Can you work these out from the model? Positions are in its coordinate system, mm. Give positions to 0.01 mm unless a question says otherwise; leave off trailing zeros. Order: outer loops, then holes, each group sorted by start corner. A loop starts at its lowest first (then second) coordinate and runs counter-clockwise, first axis right, second up. Notation, with made-up numbers: (2.5, -15.75) - (37.5, -15.75) arc R12 ccw to (37.5, -11.75) - close; hole circle Ø1 at (29, 15). An arc over 180 degrees is marked (long way). Answer as a JSON object with one key per item and string values.
```python
from build123d import *

# Parameters (mm, degrees)
CYLINDER125_R                     = 1.6
CYLINDER125_DEPTH                 = 40
CYLINDER126_R                     = 1.6
CYLINDER126_DEPTH                 = 40
EXTRUDE051_DEPTH                  = 10
SKETCH042_W                       = 4.5
SKETCH042_H                       = 27
EXTRUDE052_DEPTH                  = 21
PART_MIRRORING001_PLACEMENT_ANGLE = 180


with BuildPart() as cylinder125:
    # Cylinder125 → Cylinder125 (new body)
    with BuildSketch(Plane(origin=(5.3, 42, 40.5), x_dir=(0, 0, -1), z_dir=(0, -1, 0))):
        Circle(CYLINDER125_R)
    extrude(amount=CYLINDER125_DEPTH)


with BuildPart() as cylinder126:
    # Cylinder126 → Cylinder126 (new body)
    with BuildSketch(Plane(origin=(8.3, 42, 54.5), x_dir=(0, 0, -1), z_dir=(0, -1, 0))):
        Circle(CYLINDER126_R)
    extrude(amount=CYLINDER126_DEPTH)


with BuildPart() as extrude051:
    # Sketch041 → Extrude051 (new body)
    with BuildSketch(Plane.XZ):
        Polygon((-8.16038, 62.64716), (-8.16038, 30.419451), (4.410427, 62.64716), align=None)
    extrude(amount=-EXTRUDE051_DEPTH)


with BuildPart() as extrude051_1:
    # Extrude051 placement: moved
    add(extrude051.part.moved(Location((0, 8, 0))))


with BuildPart() as cut134:
    # Sketch042 → Extrude052 (new body)
    with BuildSketch(Plane.YZ):
        with Locations((12.25, 48.5)):
            Rectangle(SKETCH042_W, SKETCH042_H)
    extrude(amount=EXTRUDE052_DEPTH)


with BuildPart() as cut134_1:
    # Extrude052 placement: moved
    add(cut134.part.moved(Location((-7, 0, 0))))

    # Cut128: cut Extrude051
    add(extrude051_1.part, mode=Mode.SUBTRACT)


with BuildPart() as cut134_2:
    # Cut128 placement: moved
    add(cut134_1.part.moved(Location((0, -7, 0))))

    # Cut133: cut Cylinder126
    add(cylinder126.part, mode=Mode.SUBTRACT)

    # Cut134: cut Cylinder125
    add(cylinder125.part, mode=Mode.SUBTRACT)


with BuildPart() as part_mirroring001:
    # Part__Mirroring001: instance of Cut134
    add(cut134_2.part.mirror(Plane(origin=(3.813159, 4e-06, 48.5), x_dir=(1, 0, 0), z_dir=(0, 1, 0))))


with BuildPart() as part_mirroring001_1:
    # Part__Mirroring001 placement: moved
    add(part_mirroring001.part.moved(Location((237.6, 0, 0))).rotate(Axis((237.6, 0, 0), (0, 0, 1)), PART_MIRRORING001_PLACEMENT_ANGLE))


solid = part_mirroring001_1.part
```
Q1. If we section it at C-C, the plane y = 6.6: Please give me the cut outline in (x, z), then the cut area to 3 significant figures.
Recorded:
{"outline": "(223.6, 35) - (243.97, 35) - (233.44, 62) - (223.6, 62) - close; hole circle Ø3.2 at (229.3, 54.5); hole circle Ø3.2 at (232.3, 40.5)", "area": "392 mm^2"}
Q2. We'd pull the mould along X, two halves only. Please class faces 1 (the face through (232, 3, 48)), 2 (the face through (223.6, 5, 49)), 3 (the face through (227.95, 5.28, 53.64)): released by +X, released by -X, zero draft, split by the parting line, or undercut.
Recorded:
{"face 1": "zero draft", "face 2": "released by -X", "face 3": "undercut"}
Q3. I need wall thicknesses on L1, parallel to Z at x = 232.3, y = 4.85; L2, parallel to Z at x = 229.3, y = 4.1; L3, parallel to X at y = 4.05, z = 39.75. Which ranges of each line are inside material? Lowest first, please.
Recorded:
{"L1": "z = 35 to 38.9, 42.1 to 62", "L2": "z = 35 to 52.9, 56.1 to 62", "L3": "x = 223.6 to 230.89, 233.71 to 242.12"}
Q4. If we section it at D-D, the plane z = 37.25: Please give me the cut outline in (x, y).
Recorded:
{"outline": "(223.6, 3) - (243.1, 3) - (243.1, 7.5) - (223.6, 7.5) - close"}
Q5. If we section it at B-B, the plane z = 54.5: Please give me the cut outline in (x, y).
Recorded:
{"outline": "(223.6, 3) - (227.7, 3) - (227.7, 7.5) - (223.6, 7.5) - close; (230.9, 3) - (236.37, 3) - (236.37, 7.5) - (230.9, 7.5) - close"}
Q6. If we section it at A-A, the plane x = 232.3: Please give me the cut outline in (y, z).
Recorded:
{"outline": "(3, 35) - (7.5, 35) - (7.5, 38.9) - (3, 38.9) - close; (3, 42.1) - (7.5, 42.1) - (7.5, 62) - (3, 62) - close"}
